from build123d import *

# Parameters (mm, degrees)
ESQUISSE1_R          = 1.25
BOSS_EXTRU_1_DEPTH   = 0.5
D_GAGEMENT_M41_D     = 4.5
D_GAGEMENT_M41_DEPTH = 16


with BuildPart() as part:
    # Esquisse1 → Boss.-Extru.1 (new body)
    with BuildSketch(Plane.XY):
        Polygon((0, 0), (0, -50), (8, -50), (8, -10), (20, -10), (20, 0), align=None)
        with Locations((15, -5)):
            Circle(ESQUISSE1_R, mode=Mode.SUBTRACT)
        with Locations((5, -5)):
            Circle(ESQUISSE1_R, mode=Mode.SUBTRACT)
    extrude(amount=BOSS_EXTRU_1_DEPTH)

    # Dégagement M41
    with Locations(Plane.XY.offset(0.5)):
        with Locations((5, -5), (15, -5)):
            Hole(D_GAGEMENT_M41_D / 2, depth=D_GAGEMENT_M41_DEPTH)


solid = part.part
Can you work these out from the model? Positions are in its coordinate system, mm. Round coordinates to 2 decimals unless told otherwise and drop trailing zeros. Write each loop counter-clockwise with the first axis right and the second up, starting at its lowest first coordinate (ties: lowest second). Pieces come first, ordered by that corner, then holes. Notation, with made-up numbers: (50.5, 34.25) -> (56.5, 34.25) arc R13 cw to (56.5, 49.25) -> close; hole circle Ø4 at (55, 61.5). An arc over 180 degrees is marked (long way). Use one line per item in the form item = value. Start each with the question number.
Q1. Imagine slicing it at A-A (x = 15). Please give me the cut outline in (y, z), then the cut area to 3 significant figures.
Q2. Imagine slicing it at C-C (z = 0.1). Please give me the cut outline in (x, y).
Q3. I'm going to push flat-ended pins straight in: P1, Ø1, axis at x = 2.5, y = -17.5, coming from the -Z side; P2, Ø4, axis at x = 15, y = -5, coming from the +Z side (3 decimals). Where does each tip first touch, or does it pass through?
Q4. Imagine slicing it at D-D (x = 5). Please give me the cut outline in (y, z), then the cut area to 4 significant figures.
Q5. Imagine slicing it at B-B (y = -5). Please give me the cut outline in (x, z).
Q6. If I drill on probe 1 along Y at (x, z) = (5, 0.2); probe 2 along Y at (x, z) = (15, 0.3); probe 3 along X at (y, z) = (-7, 0.35), over which ranges is the centre line in solid material (lowest first)? Write a range as [from, to].
Q7. We'd pull the mould along Y, two halves only. Please class faces 1 (the face through (2.854, -4.324, 0.247)), 2 (the face through (5, -19, 0.5)): +Y half, -Y half, draft (parallel to the pull), parting line (faces both ways), or undercut.
Worked out:
q1.outline = (-10, 0) -> (-7.25, 0) -> (-7.25, 0.5) -> (-10, 0.5) -> close; (-2.75, 0) -> (0, 0) -> (0, 0.5) -> (-2.75, 0.5) -> close
q1.area = 2.75 mm^2
q2.outline = (0, -50) -> (8, -50) -> (8, -10) -> (20, -10) -> (20, 0) -> (0, 0) -> close; hole circle Ø4.5 at (5, -5); hole circle Ø4.5 at (15, -5)
q3.P1 = 0
q3.P2 = through
q4.outline = (-50, 0) -> (-7.25, 0) -> (-7.25, 0.5) -> (-50, 0.5) -> close; (-2.75, 0) -> (0, 0) -> (0, 0.5) -> (-2.75, 0.5) -> close
q4.area = 22.75 mm^2
q5.outline = (0, 0) -> (2.75, 0) -> (2.75, 0.5) -> (0, 0.5) -> close; (7.25, 0) -> (12.75, 0) -> (12.75, 0.5) -> (7.25, 0.5) -> close; (17.25, 0) -> (20, 0) -> (20, 0.5) -> (17.25, 0.5) -> close
q6.probe_1 = [-50, -7.25], [-2.75, 0]
q6.probe_2 = [-10, -7.25], [-2.75, 0]
q6.probe_3 = [0, 3.97], [6.03, 13.97], [16.03, 20]
q7.face_1 = undercut
q7.face_2 = draft
